Geometry check sheet. Reference: the model listing, model coordinates, mm. Round coordinates to 2 decimals unless told otherwise and drop trailing zeros. Write each loop counter-clockwise with the first axis right and the second up, starting at its lowest first coordinate (ties: lowest second). Pieces come first, ordered by that corner, then holes. Notation, with made-up numbers: (66.25, 11) - (113.25, 11) arc R24 cw to (113.25, 29) - close; hole circle Ø11 at (19.25, -6). An arc over 180 degrees is marked (long way). Return JSON: item names as keys, results as strings.
Autodesk Inventor part; units mm, degrees
ref_plane "YZ Plane" through (0, 0, 0) normal (1, 0, 0) x (0, 1, 0)
ref_plane "XZ Plane" through (0, 0, 0) normal (0, 1, 0) x (-1, 0, 0)
ref_plane "XY Plane" through (0, 0, 0) normal (0, 0, 1) x (1, 0, 0)
sketch "Sketch1" plane through (0, 0, 0) normal (0, 1, 0) x (-1, 0, 0)
  line L0 (0, 0) -> (-146.05, 0)
  line L1 (-146.05, 0) -> (-146.05, -231.775)
  line L2 (-146.05, -231.775) -> (0, -231.775)
  line L3 (0, -231.775) -> (0, 0)
  dimension "d0" = 146.05
  dimension "d1" = 231.775
extrude "Extrusion1" add sketch "Sketch1" along normal blind 3.175
sketch "Sketch2" plane through (146.05, 0, 0) normal (1, 0, 0) x (0, 0, -1)
  line L0 (0, 0) -> (231.775, 0)
  line L1 (231.775, 0) -> (231.775, 194.818)
  line L2 (231.775, 194.818) -> (120.65, 194.818)
  line L3 (120.65, 194.818) -> (120.65, 122.809)
  line L4 (0, 0) -> (0, 122.809)
  line L5 (0, 122.809) -> (120.65, 122.809)
  dimension "d4" = 194.818
  dimension "d5" = 111.125
  dimension "d6" = 72.009
  dimension "d7" = 122.809
extrude "Extrusion2" add sketch "Sketch2" against normal blind 3.175
sketch "Sketch3" plane through (146.05, 0, -231.775) normal (0, 0, -1) x (-1, 0, 0)
  line L0 (0, 0) -> (0, 194.818)
  line L1 (0, 194.818) -> (146.05, 194.818)
  line L2 (146.05, 194.818) -> (146.05, 0)
  line L3 (146.05, 0) -> (0, 0)
  line L4 (0, 0) -> (0, 194.818)
extrude "Extrusion3" add sketch "Sketch3" against normal blind 3.175
sketch "Sketch4" plane through (0, 0, -231.775) normal (-1, 0, 0) x (0, 0, 1)
  line L0 (231.775, 0) -> (231.775, 3.175)
  line L1 (231.775, 122.809) -> (111.125, 122.809)
  line L2 (231.775, 0) -> (200.025, 0)
  line L3 (200.025, 0) -> (200.025, 122.809)
  line L4 (200.025, 122.809) -> (231.775, 122.809)
  line L5 (231.775, 122.809) -> (231.775, 0)
  dimension "d12" = 31.75
extrude "Extrusion4" add sketch "Sketch4" against normal blind 3.175
properties part number "Shooting_Case"
(1) Section check A-A, the plane y = 67.5. Enter the section's corners in (x, z) (3 decimals).
Response values:
{"outline": "(0, -231.775) - (146.05, -231.775) - (146.05, 0) - (142.875, 0) - (142.875, -228.6) - (0, -228.6) - close; (0, -31.75) - (3.175, -31.75) - (3.175, 0) - (0, 0) - close"}
(2) Section check C-C, the plane z = -101. Enter the section's corners in (x, y) (3 decimals), plus the area to 3 significant figures.
Response values:
{"outline": "(0, 0) - (146.05, 0) - (146.05, 122.809) - (142.875, 122.809) - (142.875, 3.175) - (0, 3.175) - close", "area": "844 mm^2"}
(3) Material ranges on line 1 along Z through (x, y) = (109.5, 108) (3 decimals); line 2 along Y through (x, z) = (101.5, -201) (3 decimals); line 3 along X through (y, z) = (21.5, -88.5) (3 decimals), recorded low to high. Write a range as [from, to].
Response values:
{"line 1": "z = [-231.775, -228.6]", "line 2": "y = [0, 3.175]", "line 3": "x = [142.875, 146.05]"}
(4) Section check B-B, the plane x = 56.5. Enter the section's corners in (y, z) (3 decimals), plus the area to 3 significant figures.
Response values:
{"outline": "(0, -231.775) - (194.818, -231.775) - (194.818, -228.6) - (3.175, -228.6) - (3.175, 0) - (0, 0) - close", "area": "1,340 mm^2"}
(5) Release check for a two-part mould opening along X. For faces 1 (the face through (3.175, 64, -16)), 2 (the face through (0, 46, -31)), 3 (the face through (72, 100, -228.6)) record: pulls with the +X half, pulls with the -X half, needs draft (parallel to the pull), parting line crosses it, or undercut.
Response values:
{"face 1": "undercut", "face 2": "pulls with the -X half", "face 3": "needs draft"}
(6) Gauge pin test, flat ends, axial feed: pin 1 (3.5 mm diameter, centred on x = 2, z = -10.5, fed in from +Y); pin 2 (2.5 mm diameter, centred on x = 144, y = 167, fed in from +Z); pin 3 (12 mm diameter, centred on y = 104, z = -79, fed in from -X) (3 decimals). Record the tip position at first contact, or that the pin passes through.
Response values:
{"pin 1": "stops at y = 122.81", "pin 2": "stops at z = -120.65", "pin 3": "stops at x = 142.875"}
